The model under review builds one solid part; all positions refer to its coordinate system, in mm. Give positions to 0.01 mm unless a question says otherwise; leave off trailing zeros. Loops run counter-clockwise (first coordinate to the right, second up) from the corner with the lowest first, then second, coordinate; pieces in that order, holes last. Notation, with made-up numbers: M 36,-8 L 84,-8 A24 cw 84,6 Z; hole C 12.5,-25.75 d4. An arc over 180 degrees is marked long. Put each result on its own line as item: value. Start each with the question number.
Autodesk Inventor part; units mm, degrees
ref_plane "YZ Plane" through (0, 0, 0) normal (1, 0, 0) x (0, 1, 0)
ref_plane "XZ Plane" through (0, 0, 0) normal (0, 1, 0) x (-1, 0, 0)
ref_plane "XY Plane" through (0, 0, 0) normal (0, 0, 1) x (1, 0, 0)
sketch "Sketch1" plane through (0, 0, 0) normal (0, 0, 1) x (1, 0, 0)
  circle A0 centre (0, 0) radius 12.7
  circle A1 centre (0, 0) radius 5
  dimension "d0" = 25.4
  dimension "d1" = 10
extrude "Extrusion1" add sketch "Sketch1" along normal mid plane 200
sketch "Sketch2" plane through (0, 0, 100) normal (0, 0, 1) x (1, 0, 0)
  line L0 (-17.78, 0) -> (17.78, 0)
  line L1 (0, -17.78) -> (0, 17.78)
  circle A0 centre (0, 0) radius 8 construction
  point P0 (0, 8)
  point P1 (8, 0)
  point P2 (0, -8)
  point P3 (-8, 0)
  dimension "d4" = 16
hole "Hole1" at (0, 8, 100) at (8, 0, 100) at (0, -8, 100) at (-8, 0, 100) direction (0, 0, -1) diameter 2.459 depth 10
mirror "Mirror1" about plane through (0, 0, 0) normal (0, 0, 1) of "Hole1"
properties part number "barra solida hueca"
Item 1: To check wall thickness, follow L1, parallel to Y at x = 0, z = -93; L2, parallel to Y at x = -0.5, z = -66; L3, parallel to Y at x = 8, z = -97.25. State the ranges of each line that lie inside material, in increasing order. Write a range as [from, to].
Item 2: Clearance check with flat-ended pins moving along their axes: pin 1 Ø8 at (y, z) = (-1.5, 5) entering from -X; pin 2 Ø1 at (x, z) = (-8, 80) entering from +Y; pin 3 Ø1.5 at (x, z) = (7.5, -17.5) entering from +Y; pin 4 Ø0.7 at (x, y) = (-8, 0) entering from -Z. State where each tip first meets the part, or that it passes through.
Item 3: Draft analysis for pull direction X (two halves, no side actions). For faces 1 (the cylindrical face through (-2.75, -12.4, 1.4)), 2 (the flat face through (5.5, 0.2, 100)), 3 (the cylindrical face through (-1.08, -4.88, 1.4)), state which applies: +X half, -X half, draft (parallel to the pull), parting line (faces both ways), or undercut.
Item 4: Consider section B-B, the plane x = 3. Write out the cut boundary in (y, z), plus the area to 3 significant figures.
Item 5: Consider section A-A, the plane z = 13.5. Write out the cut boundary in (x, y).
Report:
1. L1: [-12.7, -9.23], [-6.77, -5], [5, 6.77], [9.23, 12.7]
1. L2: [-12.69, -4.97], [4.97, 12.69]
1. L3: [-9.86, -1.23], [1.23, 9.86]
2. pin 1: x = -12.7
2. pin 2: y = 10.25
2. pin 3: y = 10.76
2. pin 4: z = -90
3. face 1: parting line
3. face 2: draft
3. face 3: undercut
4. outline: M -12.34,-100 L -4,-100 L -4,100 L -12.34,100 Z; M 4,-100 L 12.34,-100 L 12.34,100 L 4,100 Z
4. area: 3,340 mm²
5. outline: C 0,0 d25.4; hole C 0,0 d10
